For this review, take the finished solid that the model builds, in its own axes (mm). Face numbers are marked on the shaded views. A direction names the side the tool comes from. Give positions to 0.01 mm unless a question says otherwise; leave off trailing zeros. Write each loop counter-clockwise with the first axis right and the second up, starting at its lowest first coordinate (ties: lowest second). Pieces come first, ordered by that corner, then holes. Notation, with made-up numbers: (-24, 35.5) -> (5, 35.5) arc R25 cw to (5, 59.5) -> close; hole circle Ø1 at (-1, -3). An arc over 180 degrees is marked (long way). Write item = value, one per line.
```python
from build123d import *

# Parameters (mm, degrees)
F1_DEPTH  = 31.75
F2_R      = 6.35
F3_DEPTH  = 31.75
F5_DEPTH  = 31.75
F7_DEPTH  = 19.05
F8_DEPTH  = 6.35
F9_W      = 12.7
F9_H      = 12.7
F10_DEPTH = 31.75
F11_W     = 12.7
F11_H     = 12.7
F12_DEPTH = 19.05
F14_DEPTH = 12.7
F15_W     = 12.7
F15_H     = 12.7
F16_DEPTH = 12.7
F18_DEPTH = 12.7
F19_R     = 1.5875
F20_DEPTH = 12.7
F22_DEPTH = 6.35


with BuildPart() as f1:
    # F0 (on Front) → F1 (new body)
    with BuildSketch(Plane.XZ):
        Polygon((-9.6981803781, 6.35), (-22.3981803781, 6.35), (-22.3981803781, 0), (28.4018196219, 0), (28.4018196219, 6.35), (15.7018196219, 6.35), (15.7018196219, 57.15), (-9.6981803781, 57.15), align=None)
    extrude(amount=F1_DEPTH)

    # F2 (on face) → F3 (cut)
    with BuildSketch(Plane.XZ.offset(31.75)):
        with Locations((3.0018196219, 44.45)):
            Circle(F2_R)
    extrude(amount=-F3_DEPTH, mode=Mode.SUBTRACT)

    # F4 (on face) → F5 (cut)
    with BuildSketch(Plane.XZ.offset(31.75)):
        with BuildLine():
            ThreePointArc((-9.6981803781, 44.45), (-5.9784365163, 53.4302561039), (3.0018195733, 57.15))
            Line((3.0018195733, 57.15), (-9.6981803781, 57.15))
            Line((-9.6981803781, 57.15), (-9.6981803781, 44.45))
        make_face()
        with BuildLine():
            ThreePointArc((3.0018195733, 57.15), (11.9820757258, 53.4302561383), (15.7018196219, 44.45))
            Line((15.7018196219, 44.45), (15.7018196219, 57.15))
            Line((15.7018196219, 57.15), (3.0018195733, 57.15))
        make_face()
    extrude(amount=-F5_DEPTH, mode=Mode.SUBTRACT)

    # F6 (on face) → F7 (cut)
    with BuildSketch(Plane.XZ.offset(31.75)):
        with BuildLine():
            Line((15.7018196219, 6.35), (15.7018196219, 44.45))
            ThreePointArc((15.7018196219, 44.45), (3.0018196219, 31.75), (-9.6981803781, 44.45))
            Line((-9.6981803781, 44.45), (-9.6981803781, 6.35))
            Line((-9.6981803781, 6.35), (15.7018196219, 6.35))
        make_face()
    extrude(amount=-F7_DEPTH, mode=Mode.SUBTRACT)

    # F8 (cut): a face of the model
    f8_faces = [f1.faces().sort_by_distance(p)[0] for p in [
        (15.3426093771, -31.75, 44.45),
    ]]
    extrude(f8_faces, amount=-F8_DEPTH, mode=Mode.SUBTRACT)

    # F9 (on face) → F10 (join)
    with BuildSketch(Plane.XZ.offset(31.75)):
        with Locations((-16.0481803781, 12.7)):
            Rectangle(F9_W, F9_H)
    extrude(amount=-F10_DEPTH)

    # F11 (on face) → F12 (cut)
    with BuildSketch(Plane.XZ.offset(31.75)):
        with Locations((-16.0481803781, 12.7)):
            Rectangle(F11_W, F11_H)
    extrude(amount=-F12_DEPTH, mode=Mode.SUBTRACT)

    # F13 (on face) → F14 (cut)
    with BuildSketch(Plane.XZ.offset(12.7)):
        with BuildLine():
            Line((-22.3981803781, 19.05), (-22.3981803781, 6.35))
            ThreePointArc((-22.3981803781, 6.35), (-13.417924257, 10.0697438789), (-9.6981803781, 19.05))
            Line((-9.6981803781, 19.05), (-22.3981803781, 19.05))
        make_face()
    extrude(amount=-F14_DEPTH, mode=Mode.SUBTRACT)

    # F15 (on face) → F16 (join)
    with BuildSketch(Plane.XZ.offset(12.7)):
        with Locations((22.0518196219, 12.7)):
            Rectangle(F15_W, F15_H)
    extrude(amount=-F16_DEPTH)

    # F17 (on face) → F18 (cut)
    with BuildSketch(Plane.XZ.offset(12.7)):
        with BuildLine():
            Line((28.4018196219, 19.05), (15.7018196219, 19.05))
            ThreePointArc((15.7018196219, 19.05), (19.4215635009, 10.0697438789), (28.4018196219, 6.35))
            Line((28.4018196219, 6.35), (28.4018196219, 19.05))
        make_face()
    extrude(amount=-F18_DEPTH, mode=Mode.SUBTRACT)

    # F19 (on face) → F20 (cut)
    with BuildSketch(Plane.XY.offset(6.35)):
        with Locations((-12.8731803781, -22.225)):
            Circle(F19_R)
        with Locations((18.8768196219, -22.225)):
            Circle(F19_R)
    extrude(amount=-F20_DEPTH, mode=Mode.SUBTRACT)

    # F21 (on face) → F22 (cut)
    with BuildSketch(Plane.XY.offset(6.35)):
        with BuildLine():
            ThreePointArc((-9.6981803781, -31.75), (-18.6784364991, -28.0302561211), (-22.3981803781, -19.05))
            Line((-22.3981803781, -19.05), (-22.3981803781, -31.75))
            Line((-22.3981803781, -31.75), (-9.6981803781, -31.75))
        make_face()
        with BuildLine():
            ThreePointArc((28.4018196219, -19.05), (24.682075743, -28.0302561211), (15.7018196219, -31.75))
            Line((15.7018196219, -31.75), (28.4018196219, -31.75))
            Line((28.4018196219, -31.75), (28.4018196219, -19.05))
        make_face()
    extrude(amount=-F22_DEPTH, mode=Mode.SUBTRACT)


solid = f1.part
```
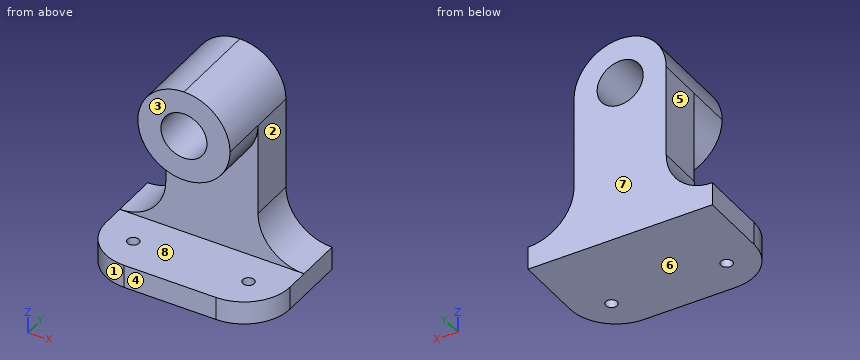
(1) For pin 1 (2 mm diameter, centred on y = -13.5, z = 25, fed in from -X); pin 2 (10 mm diameter, centred on x = 11, z = 11.5, fed in from -Y); pin 3 (5 mm diameter, centred on y = -7.5, z = 24, fed in from +X), all flat-tipped, find the tip position at first contact; note any pin that passes through.
Answers below:
pin_1 = -9.7
pin_2 = -12.7
pin_3 = 15.7
(2) Take a section at B-B (x = 8). Write out the cut boundary in (y, z).
Answers below:
outline = (-31.75, 0) -> (0, 0) -> (0, 40.53) -> (-25.4, 40.53) -> (-25.4, 32.77) -> (-12.7, 32.77) -> (-12.7, 6.35) -> (-31.75, 6.35) -> close; (-25.4, 48.37) -> (0, 48.37) -> (0, 56.13) -> (-25.4, 56.13) -> close
(3) Tool access review of the marked faces 1, 2, 3, 4 and 5: name each direction out of +Z, -Z, +X, -X, +Y, -Y from which nothing blocks a thin tool from reaching the whole face with its end or side.
Answers below:
face_1 = +Z, -Z, -X, -Y
face_2 = +Z, +X, +Y, -Y
face_3 = +Z, +X, -X, -Y
face_4 = +Z, -Z, +X, -X, -Y
face_5 = +Z, -X, +Y, -Y
(4) Take a section at A-A (y = -2). Write out the cut boundary in (x, z), plus the area to 3 significant figures.
Answers below:
outline = (-22.4, 0) -> (28.4, 0) -> (28.4, 6.35) arc R12.7 cw to (15.7, 19.05) -> (15.7, 44.45) arc R12.7 ccw to (-9.7, 44.45) -> (-9.7, 19.05) arc R12.7 cw to (-22.4, 6.35) -> close; hole circle Ø12.7 at (3, 44.45)
area = 1,490 mm^2
(5) To check wall thickness, follow probe 1 along X at (y, z) = (-8.5, 44.5); probe 2 along Z at (x, y) = (6, -16); probe 3 along Z at (x, y) = (3, -8). State the ranges of each line that lie inside material, in increasing order.
Answers below:
probe_1 = -9.7 to -3.35, 9.35 to 15.7
probe_2 = 0 to 6.35, 32.11 to 38.85, 50.05 to 56.79
probe_3 = 0 to 38.1, 50.8 to 57.15
(6) Take a section at D-D (z = 37). Write out the cut boundary in (x, y), plus the area to 3 significant figures.
Answers below:
outline = (-9.7, -12.7) -> (-7.28, -12.7) -> (-7.28, -25.4) -> (13.29, -25.4) -> (13.29, -12.7) -> (15.7, -12.7) -> (15.7, 0) -> (-9.7, 0) -> close
area = 584 mm^2
(7) The part is to be moulded in two halves that separate along Z. For the marked faces 6, 7 and 8, say which applies: released by +Z, released by -Z, zero draft, split by the parting line, or undercut.
Answers below:
face_6 = released by -Z
face_7 = zero draft
face_8 = undercut
(8) Take a section at C-C (x = -4.5). Write out the cut boundary in (y, z).
Answers below:
outline = (-31.75, 0) -> (0, 0) -> (0, 54.7) -> (-25.4, 54.7) -> (-25.4, 34.2) -> (-12.7, 34.2) -> (-12.7, 6.35) -> (-31.75, 6.35) -> close
